Design review of the part shown in the three views and the two pictorial views. Dimensions are in mm from the part's minimum x, y and z. A direction names the side the tool comes from. Coordinates: 2 decimals unless noted, no trailing zeros. Loops run counter-clockwise (first coordinate to the right, second up) from the corner with the lowest first, then second, coordinate; pieces in that order, holes last. Notation, with made-up numbers: M 19,72 L 58,72 A20 ccw 58,96 Z; hole C 61,-4.75 d10. An arc over 180 degrees is marked long. Answer as a JSON object with one key per item and string values. Group by question number.
Item 1: Insertion check: pin 1 (1.5 mm diameter, centred on x = 14, z = 2, fed in from +Y); pin 2 (2 mm diameter, centred on x = 8, z = 7.5, fed in from -Y); pin 3 (4 mm diameter, centred on x = 11, z = 5, fed in from -Y); pin 4 (4.5 mm diameter, centred on x = 11, y = 11, fed in from +Z). Each pin has a flat end and moves straight along its axis. Give the tip position at first contact, or say it passes through.
Item 2: Add section C-C (z = 1). State the section outline as (x, y) points.
Item 3: Add section A-A (x = 11). State the section outline as (y, z) points, then the cut area to 3 significant figures.
Item 4: Tool access review of the marked faces 4 and 5: name each direction out of +Z, -Z, +X, -X, +Y, -Y from which nothing blocks a thin tool from reaching the whole face with its end or side.
Item 5: Mouldability with a two-part tool opening along X and no side actions: class the marked faces 1, 2 and 3 as +X half, -X half, draft (parallel to the pull), parting line (faces both ways), or undercut.
Item 6: Add section D-D (x = 6.5). State the section outline as (y, z) points, then the cut area to 3 significant figures.
Item 7: Wall thickness on L1, parallel to Y at x = 11, z = 6.5; L2, parallel to Z at x = 14.75, y = 3.75; L3, parallel to Y at x = 12.5, z = 6: over which ranges is each line inside the solid? List them lowest first. Write a range as from..to.
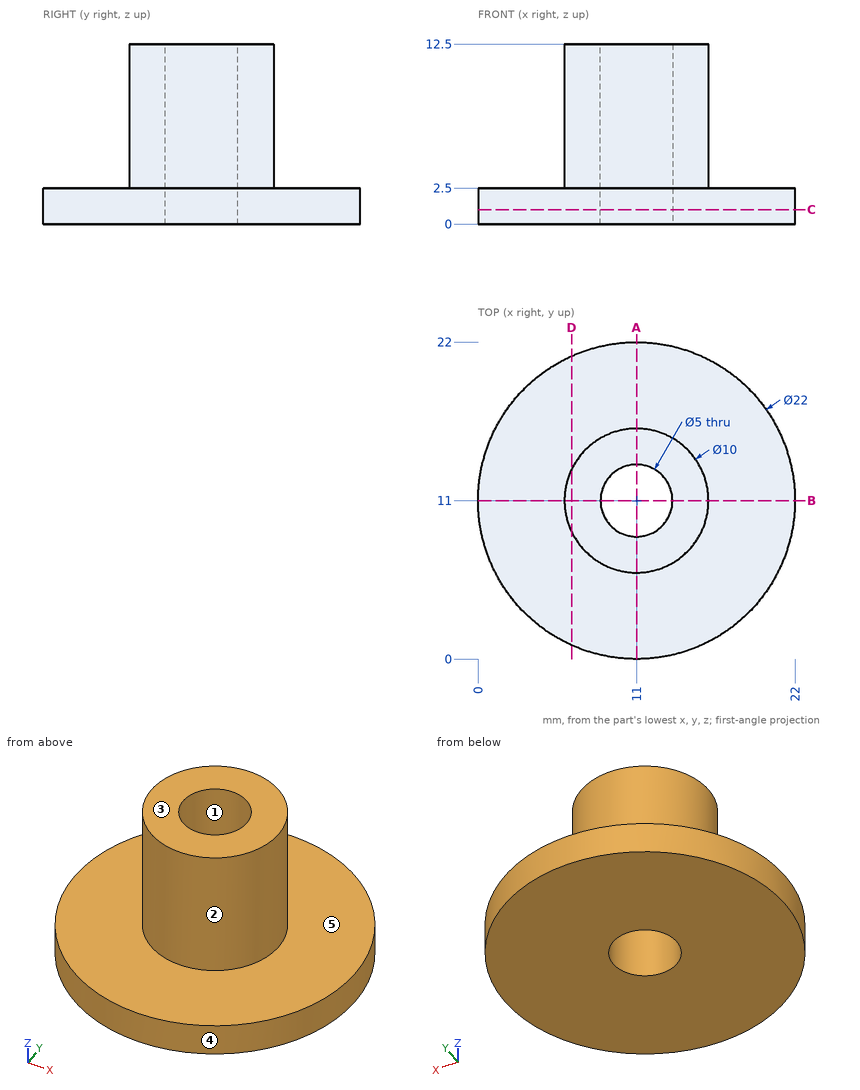
From the geometry:
{
 "1": {"pin 1": "stops at y = 21.77", "pin 2": "stops at y = 6.42", "pin 3": "stops at y = 6", "pin 4": "passes through"},
 "2": {"outline": "C 11,11 d22; hole C 11,11 d5"},
 "3": {"outline": "M 0,0 L 8.5,0 L 8.5,12.5 L 6,12.5 L 6,2.5 L 0,2.5 Z; M 13.5,0 L 22,0 L 22,2.5 L 16,2.5 L 16,12.5 L 13.5,12.5 Z", "area": "92.5 mm²"},
 "4": {"face 4": "+Z, -Z", "face 5": "+Z"},
 "5": {"face 1": "undercut", "face 2": "parting line", "face 3": "draft"},
 "6": {"outline": "M 0.96,0 L 21.04,0 L 21.04,2.5 L 13.18,2.5 L 13.18,12.5 L 8.82,12.5 L 8.82,2.5 L 0.96,2.5 Z", "area": "93.8 mm²"},
 "7": {"L1": "y = 6..8.5, 13.5..16", "L2": "z = 0..2.5", "L3": "y = 6.23..9, 13..15.77"}
}
